Part print with two shaded views. Sizes in mm from the minimum x, y, z corner. Give positions to 0.01 mm unless a question says otherwise; leave off trailing zeros. Write each loop counter-clockwise with the first axis right and the second up, starting at its lowest first coordinate (ties: lowest second). Pieces come first, ordered by that corner, then holes. Notation, with made-up numbers: (1.5, 74) -> (37.5, 74) arc R20 ccw to (37.5, 96) -> close; hole circle Ø3 at (65, 13.5). An arc over 180 degrees is marked (long way). Answer as a JSON object with one key per item and string values.
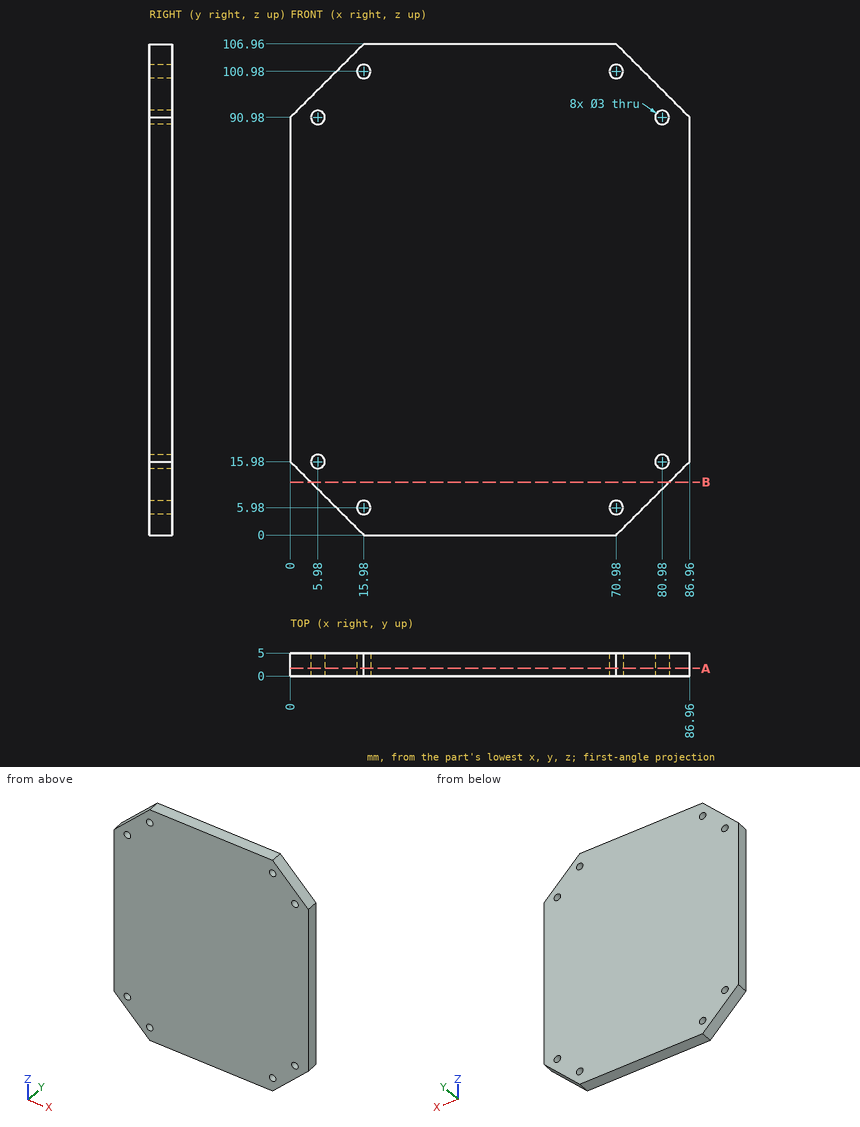
1) Slice it at A-A (y = 1.65). State how many separate pieces and enclosed holes the cut face has, then the cut area to 3 significant figures.
Model answer:
{"separate pieces": "1", "enclosed holes": "8", "area": "8,730 mm2"}
2) Slice it at B-B (z = 11.5). List the corners of the cut face in (x, y).
Model answer:
{"outline": "(4.48, 0) -> (82.48, 0) -> (82.48, 5) -> (4.48, 5) -> close"}
3) Wall check: probe 1 along Z at (x, y) = (15.5, 2.4); probe 2 along X at (y, z) = (3.6, 9); probe 3 along Z at (x, y) = (4, 3.4). Give the ranges that are in metal, low to high.
Model answer:
{"probe 1": "z = 0.48 to 4.56, 7.4 to 99.56, 102.4 to 106.48", "probe 2": "x = 6.98 to 79.98", "probe 3": "z = 11.98 to 94.98"}
